Could you check a few things on this drawing? It's one solid part, dimensions in mm from its lowest x, y, z. Give positions to 0.01 mm unless a question says otherwise; leave off trailing zeros. Order: outer loops, then holes, each group sorted by start corner. A loop starts at its lowest first (then second) coordinate and runs counter-clockwise, first axis right, second up.
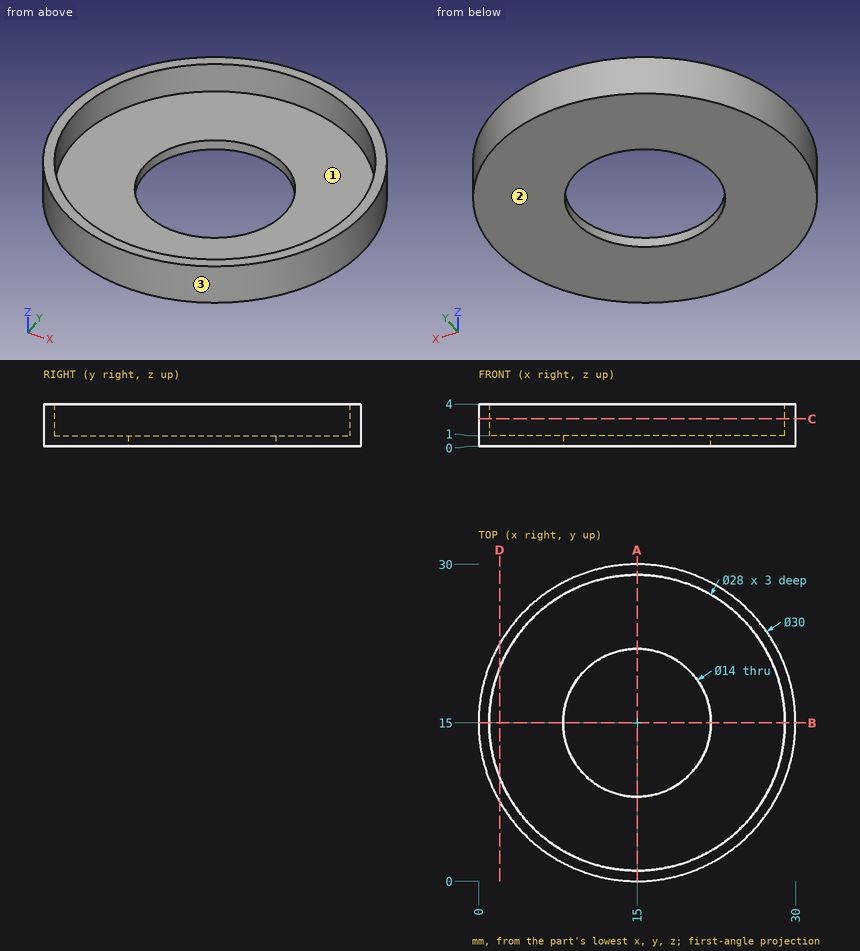
Item 1: Imagine slicing it at A-A on x = 15. List the corners of the cut face in (y, z) for me.
Findings:
outline: (0, 0) - (8, 0) - (8, 1) - (1, 1) - (1, 4) - (0, 4) - close; (22, 0) - (30, 0) - (30, 4) - (29, 4) - (29, 1) - (22, 1) - close
Item 2: Please list where these lines run through material, in increasing order: line 1 along Y through (x, z) = (15, 2.55); line 2 along Z through (x, y) = (19.75, 24.75); line 3 along Y through (x, z) = (9.25, 3.15).
Findings:
line 1: y = 0 to 1, 29 to 30
line 2: z = 0 to 1
line 3: y = 1.15 to 2.24, 27.76 to 28.85
Item 3: Imagine slicing it at D-D on x = 2. List the corners of the cut face in (y, z) for me.
Findings:
outline: (7.52, 0) - (22.48, 0) - (22.48, 4) - (20.2, 4) - (20.2, 1) - (9.8, 1) - (9.8, 4) - (7.52, 4) - close
Item 4: For pin 1 (1.5 mm diameter, centred on x = 24.5, y = 10.5, fed in from +Z); pin 2 (2 mm diameter, centred on x = 3, z = 0.5, fed in from -Y); pin 3 (1.5 mm diameter, centred on y = 21.5, z = 3, fed in from -X), each with a flat end and sliding along its axis, tell me the tip position at first contact or that it passes through.
Findings:
pin 1: stops at z = 1
pin 2: stops at y = 4.8
pin 3: stops at x = 1.15
Item 5: Imagine slicing it at C-C on z = 2.6. List the corners of the cut face in (x, y) for me.
Findings:
outline: circle Ø30 at (15, 15); hole circle Ø28 at (15, 15)
Item 6: We'd pull the mould along X, two halves only. Please class the marked faces 1, 2 and 3: +X half, -X half, draft (parallel to the pull), parting line (faces both ways), or undercut.
Findings:
face 1: undercut
face 2: draft
face 3: parting line
